Here's how the part is built. I have some questions about the finished solid (model axes, mm). A direction names the side the tool comes from. Give positions to 0.01 mm unless a question says otherwise; leave off trailing zeros. Write each loop counter-clockwise with the first axis right and the second up, starting at its lowest first coordinate (ties: lowest second). Pieces come first, ordered by that corner, then holes. Notation, with made-up numbers: (71, 56) -> (123, 56) arc R19 cw to (123, 77) -> close; hole circle Ø7 at (31.5, 46). An arc over 180 degrees is marked (long way). Answer as CSV lines item,"result". Start each with the question number.
from build123d import *

# Parameters (mm, degrees)
F0_W     = 7.9375
F0_H     = 38.1
F2_W     = 9.525
F2_H     = 9.525
F3_DEPTH = 11.1125


with BuildPart() as f1:
    # F0 (on Front) → F1 (revolve)
    with BuildSketch(Plane.XZ):
        with Locations((-25.365302, 3.109904)):
            Rectangle(F0_W, F0_H)
    revolve(axis=Axis((-21.396552, 0, 3.109904), (0, 0, -1)))

    # F2 (on face) → F3 (cut)
    with BuildSketch(Plane(origin=(0, 0, -15.940096), x_dir=(1, 0, 0), z_dir=(0, 0, -1))):
        with Locations((-21.396552, 0)):
            Rectangle(F2_W, F2_H)
    extrude(amount=-F3_DEPTH, mode=Mode.SUBTRACT)


solid = f1.part
Item 1: If we section it at B-B (z = -10): Please give me the cut outline in (x, y) (1 decimal).
Item 2: If we section it at A-A (y = 0): Please give me the cut outline in (x, z), and give its area (3 significant figures).
Item 3: I'm going to push flat-ended pins straight in: pin 1 (1.5 mm diameter, centred on x = -17.5, z = -4, fed in from -Y); pin 2 (3 mm diameter, centred on x = -19.5, z = -9.5, fed in from +Y); pin 3 (8 mm diameter, centred on y = -6, z = 14, fed in from -X). Where does each tip first touch, or does it pass through?
Item 4: If we section it at D-D (z = 1.5): Please give me the cut outline in (x, y) (1 decimal).
Item 5: If I drill on line 1 (X direction, y = 0.25, z = 5); line 2 (Z direction, x = -25, y = 0.25); line 3 (Y direction, x = -22.5, z = -10), over which ranges is the centre line in solid material (lowest first)? Write a range as [from, to].
Item 6: For faces 1 (the face through (-21, 4.762, -10)), 2 (the face through (-27, 0, -15.94)), which set-ups out of +Z, -Z, +X, -X, +Y, -Y let a thin tool reach every point of the face, with its end or its side?
Item 7: We'd pull the mould along X, two halves only. Please class faces 3 (the face through (-21, 0, -4.828)), 4 (the face through (-21, 0, 22.16)), 5 (the face through (-28.73, -3.04, 3.38)): released by +X, released by -X, zero draft, split by the parting line, or undercut.
Item 8: If we section it at C-C (x = -25.5): Please give me the cut outline in (y, z), and give its area (3 significant figures).
Final values:
1,outline,"circle Ø15.9 at (-21.4, 0); hole (-26.2, -4.8) -> (-16.6, -4.8) -> (-16.6, 4.8) -> (-26.2, 4.8) -> close"
2,outline,"(-29.33, -15.94) -> (-26.16, -15.94) -> (-26.16, -4.83) -> (-16.63, -4.83) -> (-16.63, -15.94) -> (-13.46, -15.94) -> (-13.46, 22.16) -> (-29.33, 22.16) -> close"
2,area,"499 mm2"
3,pin 1,"y = -7.29"
3,pin 2,"y = 7.93"
3,pin 3,"x = -29.08"
4,outline,"circle Ø15.9 at (-21.4, 0)"
5,line 1,"[-29.33, -13.46]"
5,line 2,"[-4.83, 22.16]"
5,line 3,"[-7.86, -4.76], [4.76, 7.86]"
6,face 1,"-Z"
6,face 2,"-Z, +X, -X, +Y, -Y"
7,face 3,"undercut"
7,face 4,"zero draft"
7,face 5,"split by the parting line"
8,outline,"(-6.79, -15.94) -> (-4.76, -15.94) -> (-4.76, -4.83) -> (4.76, -4.83) -> (4.76, -15.94) -> (6.79, -15.94) -> (6.79, 22.16) -> (-6.79, 22.16) -> close"
8,area,"412 mm2"
